from build123d import *

# Parameters (mm, degrees)
SKETCH1_R           = 3
SKETCH1_R_2         = 1.65
BOSS_EXTRUDE1_DEPTH = 2
BOSS_EXTRUDE2_START = -2
SKETCH2_R           = 5.090936199
SKETCH2_R_2         = 1.65
BOSS_EXTRUDE2_DEPTH = 2
SKETCH5_R           = 1.65
CUT_EXTRUDE1_DEPTH  = 2


with BuildPart() as part:
    # Sketch1 → Boss-Extrude1 (new body)
    with BuildSketch(Plane(origin=(0, 0, 0), x_dir=(1, 0, 0), z_dir=(0, 1, 0))):
        with BuildLine():
            Line((37.525062814, 78.755024886), (37.525062814, 32.634760232))
            ThreePointArc((37.525062814, 32.634760232), (35.515443871, 25.134760232), (30.025062814, 19.644379175))
            Line((30.025062814, 19.644379175), (29.404711739, 19.286219315))
            ThreePointArc((29.404711739, 19.286219315), (28.376391376, 18.257898952), (28, 16.853187212))
            Line((28, 16.853187212), (28, -16.853187212))
            ThreePointArc((28, -16.853187212), (28.376391376, -18.257898952), (29.404711739, -19.286219315))
            Line((29.404711739, -19.286219315), (30.025062814, -19.644379175))
            ThreePointArc((30.025062814, -19.644379175), (35.515443871, -25.134760232), (37.525062814, -32.634760232))
            Line((37.525062814, -32.634760232), (37.525062814, -78.755024886))
            ThreePointArc((37.525062814, -78.755024886), (36.943988254, -82.889585224), (35.245784257, -86.70381385))
            Line((35.245784257, -86.70381385), (26.162970632, -101.239354114))
            ThreePointArc((26.162970632, -101.239354114), (23.257062825, -103.996957657), (19.378585863, -105))
            Line((19.378585863, -105), (-19.378585863, -105))
            ThreePointArc((-19.378585863, -105), (-23.257062825, -103.996957657), (-26.162970632, -101.239354114))
            Line((-26.162970632, -101.239354114), (-35.220721442, -86.743922737))
            ThreePointArc((-35.220721442, -86.743922737), (-36.918925439, -82.929694111), (-37.5, -78.795133774))
            Line((-37.5, -78.795133774), (-37.5, -32.620290209))
            ThreePointArc((-37.5, -32.620290209), (-35.490381057, -25.120290209), (-30, -19.629909152))
            Line((-30, -19.629909152), (-29.404711739, -19.286219315))
            ThreePointArc((-29.404711739, -19.286219315), (-28.376391376, -18.257898952), (-28, -16.853187212))
            Line((-28, -16.853187212), (-28, 16.853187212))
            ThreePointArc((-28, 16.853187212), (-28.376391376, 18.257898952), (-29.404711739, 19.286219315))
            Line((-29.404711739, 19.286219315), (-30, 19.629909152))
            ThreePointArc((-30, 19.629909152), (-35.490381057, 25.120290209), (-37.5, 32.620290209))
            Line((-37.5, 32.620290209), (-37.5, 78.795133774))
            ThreePointArc((-37.5, 78.795133774), (-36.918925439, 82.929694111), (-35.220721442, 86.743922737))
            Line((-35.220721442, 86.743922737), (-26.162970632, 101.239354114))
            ThreePointArc((-26.162970632, 101.239354114), (-23.257062825, 103.996957657), (-19.378585863, 105))
            Line((-19.378585863, 105), (19.378585863, 105))
            ThreePointArc((19.378585863, 105), (23.257062825, 103.996957657), (26.162970632, 101.239354114))
            Line((26.162970632, 101.239354114), (35.245784257, 86.70381385))
            ThreePointArc((35.245784257, 86.70381385), (36.943988254, 82.889585224), (37.525062814, 78.755024886))
        make_face()
        with Locations(Location((-27.497748671, 63.999999894, 0), (0, 0, 270))):
            Circle(SKETCH1_R, mode=Mode.SUBTRACT)
        with Locations(Location((-27.498874335, 51.999999947, 0), (0, 0, 270))):
            Circle(SKETCH1_R, mode=Mode.SUBTRACT)
        with Locations(Location((-27.5, 40, 0), (0, 0, 270))):
            Circle(SKETCH1_R, mode=Mode.SUBTRACT)
        with Locations(Location((27.5, 40, 0), (0, 0, 90))):
            Circle(SKETCH1_R, mode=Mode.SUBTRACT)
        with Locations(Location((27.498874335, 51.999999947, 0), (0, 0, 90))):
            Circle(SKETCH1_R, mode=Mode.SUBTRACT)
        with Locations(Location((27.497748671, 63.999999894, 0), (0, 0, 90))):
            Circle(SKETCH1_R, mode=Mode.SUBTRACT)
        with Locations(Location((27.497748671, -63.999999894, 0), (0, 0, 270))):
            Circle(SKETCH1_R, mode=Mode.SUBTRACT)
        with Locations(Location((27.498874335, -51.999999947, 0), (0, 0, 270))):
            Circle(SKETCH1_R, mode=Mode.SUBTRACT)
        with Locations(Location((27.5, -40, 0), (0, 0, 270))):
            Circle(SKETCH1_R, mode=Mode.SUBTRACT)
        with Locations(Location((-27.5, -40, 0), (0, 0, 90))):
            Circle(SKETCH1_R, mode=Mode.SUBTRACT)
        with Locations(Location((-27.498874335, -51.999999947, 0), (0, 0, 90))):
            Circle(SKETCH1_R, mode=Mode.SUBTRACT)
        with Locations(Location((-27.497748671, -63.999999894, 0), (0, 0, 90))):
            Circle(SKETCH1_R, mode=Mode.SUBTRACT)
        with Locations(Location((-34.497748671, 71.999999894, 0), (0, 0, 270))):
            Circle(SKETCH1_R_2, mode=Mode.SUBTRACT)
        with Locations(Location((34.497748671, 71.999999894, 0), (0, 0, 90))):
            Circle(SKETCH1_R_2, mode=Mode.SUBTRACT)
        with Locations(Location((-34.497748671, -71.999999894, 0), (0, 0, 90))):
            Circle(SKETCH1_R_2, mode=Mode.SUBTRACT)
        with Locations(Location((-22.752839161, 101.035465512, 0), (0, 0, 270))):
            Circle(SKETCH1_R_2, mode=Mode.SUBTRACT)
        with Locations(Location((-33.351224445, 84.074503589, 0), (0, 0, 270))):
            Circle(SKETCH1_R_2, mode=Mode.SUBTRACT)
        with Locations(Location((-5.791877238, 90.437080228, 0), (0, 0, 270))):
            Circle(SKETCH1_R_2, mode=Mode.SUBTRACT)
        with Locations(Location((-16.390262522, 73.476118304, 0), (0, 0, 270))):
            Circle(SKETCH1_R_2, mode=Mode.SUBTRACT)
        with Locations(Location((16.390262522, 73.476118304, 0), (0, 0, 90))):
            Circle(SKETCH1_R_2, mode=Mode.SUBTRACT)
        with Locations(Location((5.791877238, 90.437080228, 0), (0, 0, 90))):
            Circle(SKETCH1_R_2, mode=Mode.SUBTRACT)
        with Locations(Location((33.351224445, 84.074503589, 0), (0, 0, 90))):
            Circle(SKETCH1_R_2, mode=Mode.SUBTRACT)
        with Locations(Location((22.752839161, 101.035465512, 0), (0, 0, 90))):
            Circle(SKETCH1_R_2, mode=Mode.SUBTRACT)
        with Locations(Location((-16.390262522, -73.476118304, 0), (0, 0, 90))):
            Circle(SKETCH1_R_2, mode=Mode.SUBTRACT)
        with Locations(Location((16.390262522, -73.476118304, 0), (0, 0, 270))):
            Circle(SKETCH1_R_2, mode=Mode.SUBTRACT)
        with Locations(Location((22.752839161, -101.035465512, 0), (0, 0, 270))):
            Circle(SKETCH1_R_2, mode=Mode.SUBTRACT)
        with Locations(Location((33.351224445, -84.074503589, 0), (0, 0, 270))):
            Circle(SKETCH1_R_2, mode=Mode.SUBTRACT)
        with Locations(Location((5.791877238, -90.437080228, 0), (0, 0, 270))):
            Circle(SKETCH1_R_2, mode=Mode.SUBTRACT)
        with Locations(Location((-5.791877238, -90.437080228, 0), (0, 0, 90))):
            Circle(SKETCH1_R_2, mode=Mode.SUBTRACT)
        with Locations(Location((-33.351224445, -84.074503589, 0), (0, 0, 90))):
            Circle(SKETCH1_R_2, mode=Mode.SUBTRACT)
        with Locations(Location((-22.752839161, -101.035465512, 0), (0, 0, 90))):
            Circle(SKETCH1_R_2, mode=Mode.SUBTRACT)
        with Locations(Location((34.497748671, -71.999999894, 0), (0, 0, 270))):
            Circle(SKETCH1_R_2, mode=Mode.SUBTRACT)
    extrude(amount=BOSS_EXTRUDE1_DEPTH)

    # Sketch2 → Boss-Extrude2 (add)
    # profile 1 of 4: a face of its own
    with BuildSketch(Plane(origin=(0, 2, 0), x_dir=(1, 0, 0), z_dir=(0, 1, 0)).offset(BOSS_EXTRUDE2_START)):
        with Locations((-34.497748671, 71.999999894)):
            Circle(SKETCH2_R)
        with Locations(Location((-34.497748671, 71.999999894, 0), (0, 0, 270))):
            Circle(SKETCH2_R_2, mode=Mode.SUBTRACT)
    # profile 2 of 4: a face of its own
    with BuildSketch(Plane(origin=(0, 2, 0), x_dir=(1, 0, 0), z_dir=(0, 1, 0)).offset(BOSS_EXTRUDE2_START)):
        with Locations((34.497748671, 71.999999894)):
            Circle(SKETCH2_R)
        with Locations(Location((34.497748671, 71.999999894, 0), (0, 0, 90))):
            Circle(SKETCH2_R_2, mode=Mode.SUBTRACT)
    # profile 3 of 4: a face of its own
    with BuildSketch(Plane(origin=(0, 2, 0), x_dir=(1, 0, 0), z_dir=(0, 1, 0)).offset(BOSS_EXTRUDE2_START)):
        with Locations((34.497748671, -71.999999894)):
            Circle(SKETCH2_R)
        with Locations(Location((34.497748671, -71.999999894, 0), (0, 0, 270))):
            Circle(SKETCH2_R_2, mode=Mode.SUBTRACT)
    # profile 4 of 4: a face of its own
    with BuildSketch(Plane(origin=(0, 2, 0), x_dir=(1, 0, 0), z_dir=(0, 1, 0)).offset(BOSS_EXTRUDE2_START)):
        with Locations((-34.497748671, -71.999999894)):
            Circle(SKETCH2_R)
        with Locations(Location((-34.497748671, -71.999999894, 0), (0, 0, 90))):
            Circle(SKETCH2_R_2, mode=Mode.SUBTRACT)
    extrude(amount=BOSS_EXTRUDE2_DEPTH)

    # Sketch5 → Cut-Extrude1 (cut)
    with BuildSketch(Plane(origin=(0, 2, 0), x_dir=(1, 0, 0), z_dir=(0, 1, 0))):
        with Locations(Location((-26.497748671, 71.999999894, 0), (0, 0, 270))):
            Circle(SKETCH5_R)
        with Locations(Location((-8, 100, 0), (0, 0, 270))):
            Circle(SKETCH5_R)
        with Locations(Location((8, 100, 0), (0, 0, 90))):
            Circle(SKETCH5_R)
        with Locations(Location((26.497748671, 71.999999894, 0), (0, 0, 90))):
            Circle(SKETCH5_R)
        with Locations(Location((26.497748671, -71.999999894, 0), (0, 0, 270))):
            Circle(SKETCH5_R)
        with Locations(Location((8, -100, 0), (0, 0, 270))):
            Circle(SKETCH5_R)
        with Locations(Location((-8, -100, 0), (0, 0, 90))):
            Circle(SKETCH5_R)
        with Locations(Location((-26.497748671, -71.999999894, 0), (0, 0, 90))):
            Circle(SKETCH5_R)
        with Locations(Location((-22.5, 30.5, 0), (0, 0, 270))):
            Circle(SKETCH5_R)
        with Locations(Location((22.5, 30.5, 0), (0, 0, 270))):
            Circle(SKETCH5_R)
        with Locations(Location((-22.5, -14.5, 0), (0, 0, 270))):
            Circle(SKETCH5_R)
        with Locations(Location((22.5, -14.5, 0), (0, 0, 270))):
            Circle(SKETCH5_R)
        with BuildLine():
            Line((-15.574688151, 66.481947499), (-15.574688151, 36.481947499))
            ThreePointArc((-15.574688151, 36.481947499), (-18.074688151, 33.981947499), (-20.574688151, 36.481947499))
            Line((-20.574688151, 36.481947499), (-20.574688151, 66.481947499))
            ThreePointArc((-20.574688151, 66.481947499), (-18.074688151, 68.981947499), (-15.574688151, 66.481947499))
        make_face()
        with BuildLine():
            Line((-17.63046279, 25), (-17.63046279, -9))
            ThreePointArc((-17.63046279, -9), (-20.13046279, -11.5), (-22.63046279, -9))
            Line((-22.63046279, -9), (-22.63046279, 25))
            ThreePointArc((-22.63046279, 25), (-20.13046279, 27.5), (-17.63046279, 25))
        make_face()
        with BuildLine():
            Line((17.63046279, 25), (17.63046279, -9))
            ThreePointArc((17.63046279, -9), (20.13046279, -11.5), (22.63046279, -9))
            Line((22.63046279, -9), (22.63046279, 25))
            ThreePointArc((22.63046279, 25), (20.13046279, 27.5), (17.63046279, 25))
        make_face()
        with BuildLine():
            Line((15.574688151, 66.481947499), (15.574688151, 36.481947499))
            ThreePointArc((15.574688151, 36.481947499), (18.074688151, 33.981947499), (20.574688151, 36.481947499))
            Line((20.574688151, 36.481947499), (20.574688151, 66.481947499))
            ThreePointArc((20.574688151, 66.481947499), (18.074688151, 68.981947499), (15.574688151, 66.481947499))
        make_face()
        with BuildLine():
            Line((15.574688151, -66.481947499), (15.574688151, -36.481947499))
            ThreePointArc((15.574688151, -36.481947499), (18.074688151, -33.981947499), (20.574688151, -36.481947499))
            Line((20.574688151, -36.481947499), (20.574688151, -66.481947499))
            ThreePointArc((20.574688151, -66.481947499), (18.074688151, -68.981947499), (15.574688151, -66.481947499))
        make_face()
        with BuildLine():
            Line((-15.574688151, -66.481947499), (-15.574688151, -36.481947499))
            ThreePointArc((-15.574688151, -36.481947499), (-18.074688151, -33.981947499), (-20.574688151, -36.481947499))
            Line((-20.574688151, -36.481947499), (-20.574688151, -66.481947499))
            ThreePointArc((-20.574688151, -66.481947499), (-18.074688151, -68.981947499), (-15.574688151, -66.481947499))
        make_face()
        Polygon((8.660254038, 49.909485966), (0, 54.909485966), (-8.660254038, 49.909485966), (-8.660254038, 39.909485966), (0, 34.909485966), (8.660254038, 39.909485966), align=None)
        Polygon((8.660254038, -44.090514034), (8.660254038, -34.090514034), (0, -29.090514034), (-8.660254038, -34.090514034), (-8.660254038, -44.090514034), (0, -49.090514034), align=None)
        Polygon((0, 62.909485966), (8.660254038, 67.909485966), (8.660254038, 77.909485966), (0, 82.909485966), (-8.660254038, 77.909485966), (-8.660254038, 67.909485966), align=None)
        Polygon((8.660254038, -62.090514034), (0, -57.090514034), (-8.660254038, -62.090514034), (-8.660254038, -72.090514034), (0, -77.090514034), (8.660254038, -72.090514034), align=None)
    extrude(amount=-CUT_EXTRUDE1_DEPTH, mode=Mode.SUBTRACT)


solid = part.part
Verification items for the finished model (mm, model axes). A direction names the side the tool comes from. Coordinates: 2 decimals unless noted, no trailing zeros. Order: outer loops, then holes, each group sorted by start corner. A loop starts at its lowest first (then second) coordinate and runs counter-clockwise, first axis right, second up. Notation, with made-up numbers: M 24,-23 L 39,-23 A14 ccw 39,-5 Z; hole C 54.25,32.25 d6. An arc over 180 degrees is marked long. One line per item, written item: value. Start each with the question number.
Item 1: Mould release check, pull along Z, two halves, no side actions. Record for faces 1 (the flat face through (-4.391, 1.014, 46.556)), 2 (the flat face through (1, 0, -1)), 3 (the cylindrical face through (23.207, 0.986, -104.024)): released by +Z, released by -Z, zero draft, split by the parting line, or undercut.
Item 2: Scan lines: probe 1 along X at (y, z) = (0.75, 14.5); probe 2 along X at (y, z) = (1.1, -40); probe 3 along X at (y, z) = (0.3, -85). Record each from-to range of solid material in increasing order.
Item 3: Sectioned sample at D-D (y = 1.15). Count the separate pieces of the cut face and the enclosed holes in it, then the cut area to 3 significant figures.
Item 4: Access from +Z, -Z, +X, -X, +Y, -Y to the whole of each face (thin tool, end or side, straight path). Record for faces 4 (the flat face through (-4.27, 1.014, -80.444)), 5 (the cylindrical face through (35.57, 0.99, -25.23)), 6 (the flat face through (-30.755, 0.986, -93.89)), 7 (the cylindrical face through (-35.545, 0.986, 25.216)), 8 (the flat face through (1, 2, -1)).
Item 5: Sectioned sample at B-B (z = 0). Enter the section's corners in (x, y), then the cut area to 3 significant figures.
Item 6: Sectioned sample at C-C (z = -52). Enter the section's corners in (x, y).
Item 7: Sectioned sample at A-A (z = 64). Enter the section's corners in (x, y).
Item 8: Gauge pin test, flat ends, axial feed: pin 1 (1 mm diameter, centred on y = 1, z = 77.5, fed in from -X); pin 2 (1 mm diameter, centred on x = -22, y = 1, fed in from -Z); pin 3 (1 mm diameter, centred on y = 0.5, z = 0.5, fed in from -X). Record the tip position at first contact, or that the pin passes through.
Conclusion:
1. face 1: undercut
1. face 2: zero draft
1. face 3: released by -Z
2. probe 1: x = -28 to -24.15, -20.85 to 20.85, 24.15 to 28
2. probe 2: x = -37.5 to -30.5, -24.5 to -20.57, -15.57 to -8.66, 8.66 to 15.57, 20.57 to 24.5, 30.5 to 37.53
2. probe 3: x = -36.16 to -34.72, -31.99 to 31.99, 34.72 to 36.16
3. separate pieces: 1
3. enclosed holes: 54
3. area: 11,600 mm^2
4. face 4: +Y, -Y
4. face 5: +X, +Y, -Y
4. face 6: -Z, -X, +Y, -Y
4. face 7: -X, +Y, -Y
4. face 8: +Z, -Z, +X, -X, +Y
5. outline: M -28,0 L -22.63,0 L -22.63,2 L -28,2 Z; M -17.63,0 L 17.63,0 L 17.63,2 L -17.63,2 Z; M 22.63,0 L 28,0 L 28,2 L 22.63,2 Z
5. area: 92.0 mm^2
6. outline: M -37.5,0 L -30.5,0 L -30.5,2 L -37.5,2 Z; M -24.5,0 L -20.57,0 L -20.57,2 L -24.5,2 Z; M -15.57,0 L -5.04,0 L -5.04,2 L -15.57,2 Z; M 5.04,0 L 15.57,0 L 15.57,2 L 5.04,2 Z; M 20.57,0 L 24.5,0 L 24.5,2 L 20.57,2 Z; M 30.5,0 L 37.53,0 L 37.53,2 L 30.5,2 Z
7. outline: M -37.5,0 L -30.5,0 L -30.5,2 L -37.5,2 Z; M -24.5,0 L -20.57,0 L -20.57,2 L -24.5,2 Z; M -15.57,0 L -8.66,0 L -8.66,2 L -15.57,2 Z; M 8.66,0 L 15.57,0 L 15.57,2 L 8.66,2 Z; M 20.57,0 L 24.5,0 L 24.5,2 L 20.57,2 Z; M 30.5,0 L 37.53,0 L 37.53,2 L 30.5,2 Z
8. pin 1: stops at x = -37.5
8. pin 2: stops at z = -104.71
8. pin 3: stops at x = -28
